Can you work these out from the model? Positions are in its coordinate system, mm. A direction names the side the tool comes from. Round coordinates to 2 decimals unless told otherwise and drop trailing zeros. Loops run counter-clockwise (first coordinate to the right, second up) from the corner with the lowest first, then second, coordinate; pieces in that order, holes last. Notation, with made-up numbers: (25, -4.75) -> (45, -4.75) arc R15 ccw to (45, 16.25) -> close; hole circle Ø2 at (85.5, 53.5). An arc over 180 degrees is marked (long way). Use a Markdown table: item, result.
from build123d import *

# Parameters (mm, degrees)
SKETCH1_R           = 2.5
BOSS_EXTRUDE2_DEPTH = 3


with BuildPart() as part:
    # Sketch1 → Boss-Extrude2 (new body)
    with BuildSketch(Plane(origin=(0, 0, 0), x_dir=(1, 0, 0), z_dir=(0, 1, 0))):
        with BuildLine():
            Line((-19.356020942, 9), (6.643979058, 9))
            ThreePointArc((6.643979058, 9), (15.643979058, 0), (6.643979058, -9))
            Line((6.643979058, -9), (-19.356020942, -9))
            Line((-19.356020942, -9), (-19.356020942, 9))
        make_face()
        with Locations(Location((-6.856020942, 0, 0), (0, 0, 270))):
            Circle(SKETCH1_R, mode=Mode.SUBTRACT)
        with BuildLine():
            Line((-6.856020942, -6.5), (6.643979058, -6.5))
            ThreePointArc((6.643979058, -6.5), (7.893979058, -5.25), (6.643979058, -4))
            Line((6.643979058, -4), (-6.856020942, -4))
            ThreePointArc((-6.856020942, -4), (-10.856020942, 0), (-6.856020942, 4))
            Line((-6.856020942, 4), (6.643979058, 4))
            ThreePointArc((6.643979058, 4), (7.893979058, 5.25), (6.643979058, 6.5))
            Line((6.643979058, 6.5), (-6.856020942, 6.5))
            ThreePointArc((-6.856020942, 6.5), (-13.356020942, 0), (-6.856020942, -6.5))
        make_face(mode=Mode.SUBTRACT)
    extrude(amount=BOSS_EXTRUDE2_DEPTH)


solid = part.part
1. Will this pin go through, and if not, where does the flat tip stop? pin 1 Ø3 at (x, z) = (-6.86, 0) entering from +Y.
Answer sheet:
| item | result |
|---|---|
| pin 1 | passes through |
2. I need wall thicknesses on line 1 (X direction, y = 0.75, z = 0); line 2 (Z direction, x = -1.5, y = 1.25); line 3 (Z direction, x = -7, y = 2.5). Which ranges of each line are inside material? Lowest first, please.
Answer sheet:
| item | result |
|---|---|
| line 1 | x = -19.36 to -13.36, -10.86 to -9.36, -4.36 to 15.64 |
| line 2 | z = -9 to -6.5, -4 to 4, 6.5 to 9 |
| line 3 | z = -9 to -6.5, -4 to -2.5, 2.5 to 4, 6.5 to 9 |
3. I want a section at C-C (x = 3). Please give me the cut outline in (y, z), plus the area to 3 significant figures.
Answer sheet:
| item | result |
|---|---|
| outline | (0, -9) -> (3, -9) -> (3, -6.5) -> (0, -6.5) -> close; (0, -4) -> (3, -4) -> (3, 4) -> (0, 4) -> close; (0, 6.5) -> (3, 6.5) -> (3, 9) -> (0, 9) -> close |
| area | 39.0 mm² |
4. Which directions (+Z, -Z, +X, -X, +Y, -Y) give clear straight access to the entire face, cutting with the end or side of a thin tool? Please do faces 1 (the flat face through (0, 1, -6.5)), 2 (the flat face through (-6, 1, 9)).
Answer sheet:
| item | result |
|---|---|
| face 1 | +Y, -Y |
| face 2 | +Z, +X, -X, +Y, -Y |
5. I want a section at A-A (z = 0). Please give me the cut outline in (x, y).
Answer sheet:
| item | result |
|---|---|
| outline | (-19.36, 0) -> (-13.36, 0) -> (-13.36, 3) -> (-19.36, 3) -> close; (-10.86, 0) -> (-9.36, 0) -> (-9.36, 3) -> (-10.86, 3) -> close; (-4.36, 0) -> (15.64, 0) -> (15.64, 3) -> (-4.36, 3) -> close |
6. I want a section at D-D (z = 5.25). Please give me the cut outline in (x, y).
Answer sheet:
| item | result |
|---|---|
| outline | (-19.36, 0) -> (-10.69, 0) -> (-10.69, 3) -> (-19.36, 3) -> close; (7.89, 0) -> (13.95, 0) -> (13.95, 3) -> (7.89, 3) -> close |
7. I want a section at B-B (y = 1.6). Please give me the cut outline in (x, z).
Answer sheet:
| item | result |
|---|---|
| outline | (-19.36, -9) -> (6.64, -9) arc R9 ccw to (6.64, 9) -> (-19.36, 9) -> close; hole circle Ø5 at (-6.86, 0); hole (-6.86, -6.5) -> (6.64, -6.5) arc R1.25 ccw to (6.64, -4) -> (-6.86, -4) arc R4 cw to (-6.86, 4) -> (6.64, 4) arc R1.25 ccw to (6.64, 6.5) -> (-6.86, 6.5) arc R6.5 ccw to start |
8. If we mould it in two halves opening along X, with no side actions, what happens to faces 3 (the flat face through (0, 1, -4)), 4 (the cylindrical face through (-13.354, 1.479, -0.143)), 5 (the flat face through (-19.356, 1, 0)), 6 (the flat face through (-2, 0, 0))? For each: +X half, -X half, draft (parallel to the pull), parting line (faces both ways), or undercut.
Answer sheet:
| item | result |
|---|---|
| face 3 | undercut |
| face 4 | undercut |
| face 5 | -X half |
| face 6 | draft |
